Part model, mm, in its own coordinate system. A direction names the side the tool comes from. Coordinates: 2 decimals unless noted, no trailing zeros. Loops run counter-clockwise (first coordinate to the right, second up) from the corner with the lowest first, then second, coordinate; pieces in that order, holes last. Notation, with made-up numbers: M -4.75,7 L 27.25,7 A13 ccw 27.25,18 Z; hole C -14,14.5 d2. An arc over 180 degrees is marked long. Answer as a JSON object with one key per item and string values. Group by question number.
1. Drill centre lines: L1, parallel to Z at x = 1371, y = 560; L2, parallel to Y at x = 529, z = -807.5; L3, parallel to Y at x = 979.5, z = 3. Where is each one in solid material? Low to high.
2. Mould opens along Y. For faces 1 (the face through (45, 570, -410)), 2 (the face through (764, 0, -15)), 3 (the face through (1490, 45, -889)) say: released by +Y, released by -Y, zero draft, split by the parting line, or undercut.
3. Saw through at A-A on y = 100.5. Write the cut outline in (x, z).
4. 3-axis set-ups, long thin cutter, end or side, ignore diameter. For faces 4 (the face through (1520, 316, -829)), 5 (the face through (440, 600, -829)), 6 (the face through (1505, 60, -889)), 7 (the face through (60, 45, -410)): which of +Z, -Z, +X, -X, +Y, -Y reach the whole face in a straight line?
5. Drop flat-ended pins along their axis: pin 1 Ø15 at (x, z) = (42, -908.5) entering from -Y; pin 2 Ø15 at (x, z) = (1501, -270.5) entering from +Y; pin 3 Ø6 at (x, y) = (809, 98.5) entering from +Z. Give the stop position or say it passes through.
6. Saw through at D-D on y = 627. Write the cut outline in (x, z).
7. Saw through at C-C on z = -366. Write the cut outline in (x, y), then the cut area to 3 significant figures.
8. Saw through at B-B on x = 812.5. Write the cut outline in (y, z).
from build123d import *

# Parameters (mm, degrees)
F1_DEPTH = 1550
F2_W     = 30
F2_H     = 30
F3_DEPTH = 920
F4_W     = 570
F4_H     = 30
F5_DEPTH = 1490


with BuildPart() as f1:
    # F0 (on Right) → F1 (new body)
    with BuildSketch(Plane.YZ):
        Polygon((680, 0), (0, 0), (0, -30), (700, -30), (700, 50), (680, 50), align=None)
    extrude(amount=F1_DEPTH)

    # F2 (on face) → F3 (join)
    with BuildSketch(Plane(origin=(0, 0, -30), x_dir=(1, 0, 0), z_dir=(0, 0, -1))):
        with Locations((1505, -45)):
            Rectangle(F2_W, F2_H)
        with Locations((1505, -585)):
            Rectangle(F2_W, F2_H)
        with Locations((45, -585)):
            Rectangle(F2_W, F2_H)
        with Locations((45, -45)):
            Rectangle(F2_W, F2_H)
    extrude(amount=F3_DEPTH)

    # F4 (on face) → F5 (join, through all)
    with BuildSketch(Plane.YZ.offset(1520)):
        with Locations((315, -815)):
            Rectangle(F4_W, F4_H)
    extrude(amount=-F5_DEPTH)


solid = f1.part
Outcome:
{
 "1": {"L1": "z = -830 to -800, -30 to 0", "L2": "y = 30 to 600", "L3": "y = 680 to 700"},
 "2": {"face 1": "undercut", "face 2": "released by -Y", "face 3": "zero draft"},
 "3": {"outline": "M 0,-30 L 1550,-30 L 1550,0 L 0,0 Z; M 30,-830 L 1520,-830 L 1520,-800 L 30,-800 Z"},
 "4": {"face 4": "-Z, +X, +Y, -Y", "face 5": "-Z, +X, -X, +Y", "face 6": "-Z, +X, -X", "face 7": "+Y, -Y"},
 "5": {"pin 1": "stops at y = 30", "pin 2": "stops at y = 600", "pin 3": "stops at z = 0"},
 "6": {"outline": "M 0,-30 L 1550,-30 L 1550,0 L 0,0 Z"},
 "7": {"outline": "M 30,30 L 60,30 L 60,60 L 30,60 Z; M 30,570 L 60,570 L 60,600 L 30,600 Z; M 1490,30 L 1520,30 L 1520,60 L 1490,60 Z; M 1490,570 L 1520,570 L 1520,600 L 1490,600 Z", "area": "3,600 mm²"},
 "8": {"outline": "M 0,-30 L 700,-30 L 700,50 L 680,50 L 680,0 L 0,0 Z; M 30,-830 L 600,-830 L 600,-800 L 30,-800 Z"}
}
